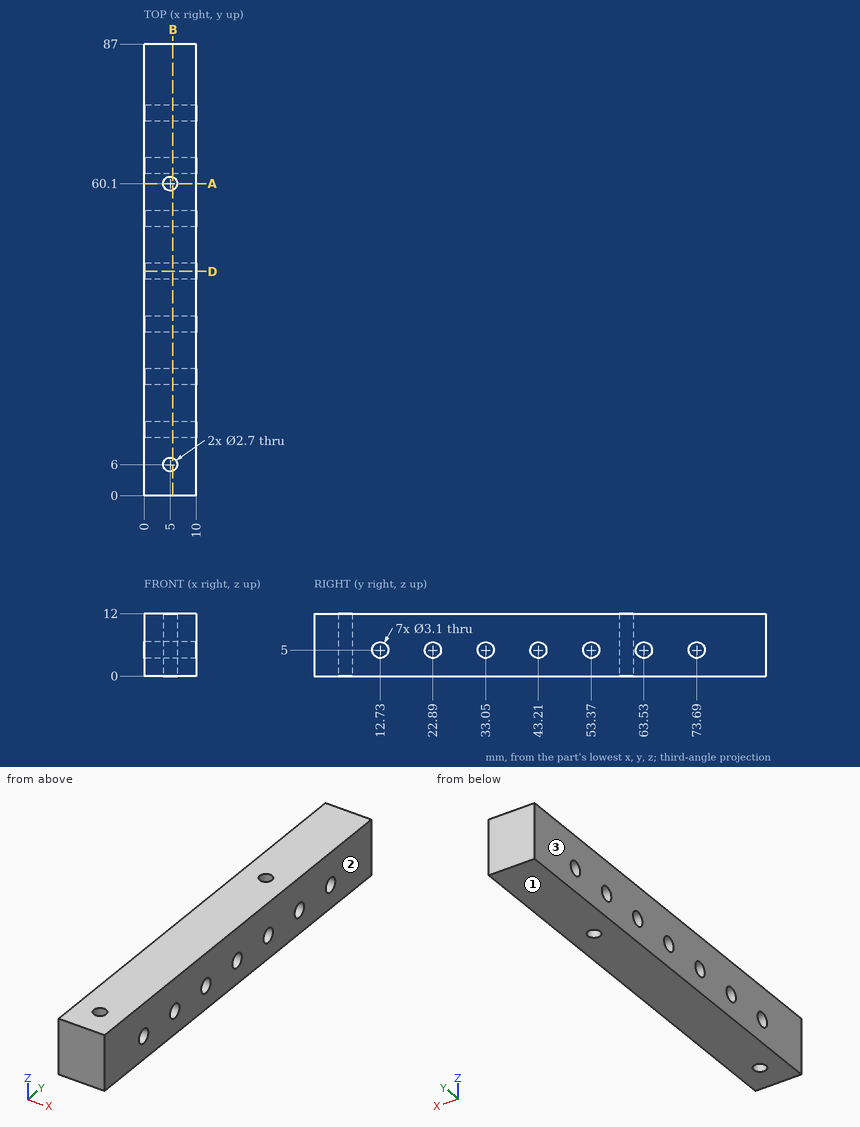
Part print with two shaded views. Sizes in mm from the minimum x, y, z corner. Coordinates: 2 decimals unless noted, no trailing zeros. Write each loop counter-clockwise with the first axis right and the second up, starting at its lowest first coordinate (ties: lowest second). Pieces come first, ordered by that corner, then holes. Notation, with made-up numbers: (26, 61) - (80, 61) arc R20 cw to (80, 87) - close; hole circle Ø6 at (28.5, 52.25). An arc over 180 degrees is marked (long way). Use a Markdown table: item, result. Add a question column.
Item 1: Two-plate mould, pull along X, no slides. Class the marked faces 1, 2 and 3: pulls with the +X half, pulls with the -X half, needs draft (parallel to the pull), parting line crosses it, or undercut.
Item 2: Drill centre lines: line 1 along Y through (x, z) = (5.5, 8); line 2 along Y through (x, z) = (4, 3); line 3 along X through (y, z) = (60.5, 2.75). Where is each one in solid material? Low to high.
Item 3: Band-saw the part on A-A, the plane y = 60.1. Write the cut outline in (x, z), and give its area (3 significant figures).
Item 4: Band-saw the part on B-B, the plane x = 5.5. Give the number of separate pieces and of enclosed holes in the cut face, and give its area (3 significant figures).
Item 5: Band-saw the part on D-D, the plane y = 43.21. Write the cut outline in (x, z), and give its area (3 significant figures).
Item 6: Drop a flat-ended pin along its axis: pin 1 (3 mm diameter, centred on y = 63.53, z = 5, fed in from -X). Give the stop position or say it passes through.
A:
| question | item | result |
|---|---|---|
| 1 | face 1 | needs draft |
| 1 | face 2 | pulls with the +X half |
| 1 | face 3 | pulls with the -X half |
| 2 | line 1 | y = 0 to 4.75, 7.25 to 58.85, 61.35 to 87 |
| 2 | line 2 | y = 0 to 5.09, 6.91 to 59.19, 61.01 to 87 |
| 2 | line 3 | x = 0 to 3.71, 6.29 to 10 |
| 3 | outline | (0, 0) - (3.65, 0) - (3.65, 12) - (0, 12) - close; (6.35, 0) - (10, 0) - (10, 12) - (6.35, 12) - close |
| 3 | area | 87.6 mm² |
| 4 | separate pieces | 3 |
| 4 | enclosed holes | 7 |
| 4 | area | 931 mm² |
| 5 | outline | (0, 0) - (10, 0) - (10, 3.45) - (0, 3.45) - close; (0, 6.55) - (10, 6.55) - (10, 12) - (0, 12) - close |
| 5 | area | 89.0 mm² |
| 6 | pin 1 | passes through |
